from build123d import *

# Parameters (mm, degrees)
SKETCH1_W           = 165
SKETCH1_H           = 95
BOSS_EXTRUDE1_DEPTH = 5
SKETCH2_W           = 155
SKETCH2_H           = 85
SKETCH2_W_2         = 145
SKETCH2_H_2         = 75
BOSS_EXTRUDE2_DEPTH = 5
SKETCH3_R           = 1.5
CUT_EXTRUDE1_DEPTH  = 5


with BuildPart() as part:
    # Sketch1 → Boss-Extrude1 (new body)
    with BuildSketch(Plane(origin=(0, 0, 0), x_dir=(1, 0, 0), z_dir=(0, 1, 0))):
        Rectangle(SKETCH1_W, SKETCH1_H)
    extrude(amount=BOSS_EXTRUDE1_DEPTH)

    # Sketch2 → Boss-Extrude2 (add)
    with BuildSketch(Plane(origin=(0, 5, 0), x_dir=(1, 0, 0), z_dir=(0, 1, 0))):
        Rectangle(SKETCH2_W, SKETCH2_H)
        Rectangle(SKETCH2_W_2, SKETCH2_H_2, mode=Mode.SUBTRACT)
    extrude(amount=BOSS_EXTRUDE2_DEPTH)

    # Sketch3 → Cut-Extrude1 (cut)
    with BuildSketch(Plane(origin=(0, 5, 0), x_dir=(1, 0, 0), z_dir=(0, 1, 0))):
        with Locations(Location((-53.973401438, 17.572735352, 0), (0, 0, 270))):
            Circle(SKETCH3_R)
        with Locations(Location((-43.973401438, 17.572735352, 0), (0, 0, 270))):
            Circle(SKETCH3_R)
        with Locations(Location((-33.973401438, 17.572735352, 0), (0, 0, 270))):
            Circle(SKETCH3_R)
        with Locations(Location((-43.973401438, 7.572735352, 0), (0, 0, 270))):
            Circle(SKETCH3_R)
        with Locations(Location((-33.973401438, 7.572735352, 0), (0, 0, 270))):
            Circle(SKETCH3_R)
        with Locations(Location((-43.973401438, -2.427264648, 0), (0, 0, 270))):
            Circle(SKETCH3_R)
        with Locations(Location((-33.973401438, -2.427264648, 0), (0, 0, 270))):
            Circle(SKETCH3_R)
        with Locations(Location((-53.973401438, 7.572735352, 0), (0, 0, 270))):
            Circle(SKETCH3_R)
        with Locations(Location((-53.973401438, -2.427264648, 0), (0, 0, 270))):
            Circle(SKETCH3_R)
    extrude(amount=-CUT_EXTRUDE1_DEPTH, mode=Mode.SUBTRACT)


solid = part.part
Check sheet for the modelled part. Datum: model origin and axes. Units: mm. A direction names the side the tool comes from. Give positions to 0.01 mm unless a question says otherwise; leave off trailing zeros. Write each loop counter-clockwise with the first axis right and the second up, starting at its lowest first coordinate (ties: lowest second). Pieces come first, ordered by that corner, then holes. Notation, with made-up numbers: (-3.75, -10.75) -> (46.25, -10.75) arc R27 cw to (46.25, 10.25) -> close; hole circle Ø6 at (10.25, 52.25). An arc over 180 degrees is marked (long way). One line per item, written item: value. Start each with the question number.
Item 1: Section check A-A on y = 8.5. Record the cut outline in (x, z), then the cut area to 3 significant figures.
Item 2: Section check D-D on z = 39.5. Record the cut outline in (x, y), then the cut area to 3 significant figures.
Item 3: Gauge pin test, flat ends, axial feed: pin 1 (3.5 mm diameter, centred on x = -33.97, z = -17.57, fed in from -Y); pin 2 (2.5 mm diameter, centred on x = -17, y = 8, fed in from +Z); pin 3 (1.5 mm diameter, centred on x = 30, y = 7, fed in from -Z); pin 4 (1.8 mm diameter, centred on x = -53.97, z = -17.57, fed in from +Y). Record the tip position at first contact, or that the pin passes through.
Item 4: Material ranges on probe 1 along X at (y, z) = (2.5, -17.5); probe 2 along X at (y, z) = (7.5, -8); probe 3 along Z at (x, y) = (-32, 8.5), recorded low to high. Write a range as from..to.
Item 5: Section check B-B on z = 14. Record the cut outline in (x, y), then the cut area to 3 significant figures.
Item 6: Tool access check on faces 5 (the cylindrical face through (-43.523, 2.535, -16.142)), 6 (the flat face through (-77.5, 7, 1)), 7 (the flat face through (-1, 7, 37.5)), 8 (the flat face through (-1, 7, -42.5)), 9 (the flat face through (82.5, 2, 1)). Record the directions out of +Z, -Z, +X, -X, +Y, -Y that give a thin tool (end or side, any length) a straight path to the whole face; none if there is none.
Item 7: Draft check along X on faces 1 (the flat face through (77.5, 7, 1)), 2 (the cylindrical face through (-52.486, 2.535, 2.232)), 3 (the flat face through (-82.5, 2, 1)), 4 (the flat face through (72.5, 7, 1)). Enter one of: +X half, -X half, draft (parallel to the pull), parting line (faces both ways), or undercut.
Item 8: Section check C-C on x = -28. Record the cut outline in (y, z), then the cut area to 3 significant figures.
Results list:
1. outline: (-77.5, -42.5) -> (77.5, -42.5) -> (77.5, 42.5) -> (-77.5, 42.5) -> close; hole (-72.5, -37.5) -> (72.5, -37.5) -> (72.5, 37.5) -> (-72.5, 37.5) -> close
1. area: 2,300 mm²
2. outline: (-82.5, 0) -> (82.5, 0) -> (82.5, 5) -> (77.5, 5) -> (77.5, 10) -> (-77.5, 10) -> (-77.5, 5) -> (-82.5, 5) -> close
2. area: 1,600 mm²
3. pin 1: y = 0
3. pin 2: z = 42.5
3. pin 3: z = -42.5
3. pin 4: through
4. probe 1: -82.5..-55.47, -52.48..-45.47, -42.48..-35.47, -32.48..82.5
4. probe 2: -77.5..-72.5, 72.5..77.5
4. probe 3: -42.5..-37.5, 37.5..42.5
5. outline: (-82.5, 0) -> (82.5, 0) -> (82.5, 5) -> (77.5, 5) -> (77.5, 10) -> (72.5, 10) -> (72.5, 5) -> (-72.5, 5) -> (-72.5, 10) -> (-77.5, 10) -> (-77.5, 5) -> (-82.5, 5) -> close
5. area: 875 mm²
6. face 5: +Y, -Y
6. face 6: +Z, -Z, -X, +Y
6. face 7: +Y
6. face 8: -Z, +X, -X, +Y
6. face 9: +Z, -Z, +X, +Y, -Y
7. face 1: +X half
7. face 2: undercut
7. face 3: -X half
7. face 4: undercut
8. outline: (0, -47.5) -> (5, -47.5) -> (5, -42.5) -> (10, -42.5) -> (10, -37.5) -> (5, -37.5) -> (5, 37.5) -> (10, 37.5) -> (10, 42.5) -> (5, 42.5) -> (5, 47.5) -> (0, 47.5) -> close
8. area: 525 mm²
